Design review of the part shown in the three views and the two pictorial views. Dimensions are in mm from the part's minimum x, y and z. A direction names the side the tool comes from. Give positions to 0.01 mm unless a question says otherwise; leave off trailing zeros. Loops run counter-clockwise (first coordinate to the right, second up) from the corner with the lowest first, then second, coordinate; pieces in that order, holes last.
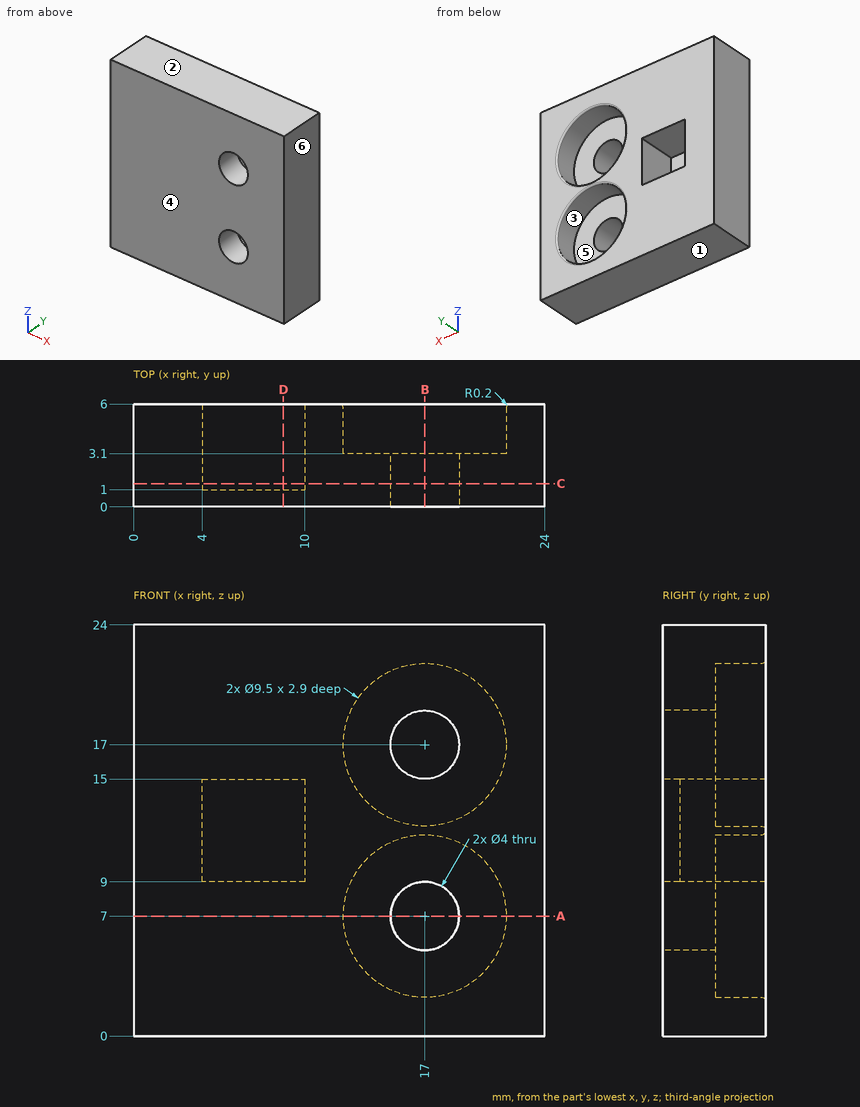
Q1. Consider section D-D on x = 8.75. Give the boundary of the cut face in (y, z), plus the area to 3 significant figures.
Answers:
outline: (0, 0) - (6, 0) - (6, 9) - (1, 9) - (1, 15) - (6, 15) - (6, 24) - (0, 24) - close
area: 114 mm2
Q2. Consider section B-B on x = 17. Give the boundary of the cut face in (y, z), plus the area to 3 significant figures.
Answers:
outline: (0, 0) - (6, 0) - (6, 2.05) arc R0.2 ccw to (5.8, 2.25) - (3.1, 2.25) - (3.1, 5) - (0, 5) - close; (0, 9) - (3.1, 9) - (3.1, 11.75) - (5.8, 11.75) arc R0.2 ccw to (6, 11.95) - (6, 12.05) arc R0.2 ccw to (5.8, 12.25) - (3.1, 12.25) - (3.1, 15) - (0, 15) - close; (0, 19) - (3.1, 19) - (3.1, 21.75) - (5.8, 21.75) arc R0.2 ccw to (6, 21.95) - (6, 24) - (0, 24) - close
area: 64.1 mm2
Q3. Machinability: for the marked faces 5 and 6, which of the approach directions +Z, -Z, +X, -X, +Y, -Y give a long, thin tool a straight path to every point of the face, cutting with its end or side? Answer none if there is none.
Answers:
face 5: +Y
face 6: +Z, -Z, +X, +Y, -Y
Q4. Mouldability with a two-part tool opening along Z and no side actions: class the marked faces 1, 2, 3 and 4 as +Z half, -Z half, draft (parallel to the pull), parting line (faces both ways), or undercut.
Answers:
face 1: -Z half
face 2: +Z half
face 3: undercut
face 4: draft
Q5. Consider section C-C on y = 1.35. Give the boundary of the cut face in (x, z), plus the area to 3 significant figures.
Answers:
outline: (0, 0) - (24, 0) - (24, 24) - (0, 24) - close; hole (4, 9) - (10, 9) - (10, 15) - (4, 15) - close; hole circle Ø4 at (17, 7); hole circle Ø4 at (17, 17)
area: 515 mm2
Q6. For pin 1 Ø3 at (x, y) = (12, 2) entering from -Z; pin 2 Ø3 at (x, z) = (17, 8) entering from +Y; pin 3 Ø3.5 at (x, z) = (17, 7) entering from -Y, all flat-tipped, find the tip position at first contact; note any pin that passes through.
Answers:
pin 1: stops at z = 0
pin 2: stops at y = 3.1
pin 3: passes through
Q7. Consider section A-A on z = 7. Give the boundary of the cut face in (x, y).
Answers:
outline: (0, 0) - (15, 0) - (15, 3.1) - (12.25, 3.1) - (12.25, 5.8) arc R0.2 ccw to (12.05, 6) - (0, 6) - close; (19, 0) - (24, 0) - (24, 6) - (21.95, 6) arc R0.2 ccw to (21.75, 5.8) - (21.75, 3.1) - (19, 3.1) - close
Q8. For probe 1 along Z at (x, y) = (17, 1.85); probe 2 along X at (y, z) = (1.65, 11.5); probe 3 along X at (y, z) = (4.15, 17), list the stretches that pass through material, from the lowest coordinate up.
Answers:
probe 1: z = 0 to 5, 9 to 15, 19 to 24
probe 2: x = 0 to 4, 10 to 24
probe 3: x = 0 to 12.25, 21.75 to 24
